Can you work these out from the model? Positions are in its coordinate system, mm. Coordinates: 2 decimals unless noted, no trailing zeros. Write each question's results on one line, items separated by ' | '. Start each with the question number.
```python
from build123d import *
from build123d.topology import SkipClean

# Parameters (mm, degrees)
SKETCH3_R               = 3.175
SKETCH3_R_2             = 1.5875
BOSS_EXTRUDE1_DEPTH     = 127
LPATTERN1_COUNT         = 2
LPATTERN1_PITCH         = 6.6675
BOSS_EXTRUDE2_DEPTH     = 127
CUT_EXTRUDE1_DEPTH      = 128.223842042
CUT_EXTRUDE1_DEPTH_BACK = 128.223842042


with BuildPart() as part:
    # Sketch3 → Boss-Extrude1 (new, symmetric)
    with BuildSketch(Plane(origin=(0, 0, 0), x_dir=(0, 0, -1), z_dir=(1, 0, 0))):
        with Locations((3.33375, 0)):
            Circle(SKETCH3_R)
        with Locations((3.33375, 0)):
            Circle(SKETCH3_R_2, mode=Mode.SUBTRACT)
    extrude(amount=BOSS_EXTRUDE1_DEPTH, both=True)


with BuildPart() as lpattern1_1:
    # LPattern1: pattern copy
    add(part.part.moved(Location(Vector(0, 0, 1) * (1 * LPATTERN1_PITCH))))


with BuildPart() as part_1:
    add(part.part)

    add(lpattern1_1.part)  # Boss-Extrude2 merges LPattern1_1
    # Sketch4 → Boss-Extrude2 (add, symmetric)
    with BuildSketch(Plane(origin=(0, 0, 0), x_dir=(0, 0, -1), z_dir=(1, 0, 0))):
        with BuildLine():
            Line((6.588125, 0.238125), (6.746875, 0.238125))
            ThreePointArc((6.746875, 0.238125), (6.811551474, 0.262993637), (6.842905738, 0.324786885))
            Line((6.842905738, 0.324786885), (6.842905738, -0.324786885))
            ThreePointArc((6.842905738, -0.324786885), (6.811551474, -0.262993637), (6.746875, -0.238125))
            Line((6.746875, -0.238125), (6.588125, -0.238125))
            ThreePointArc((6.588125, -0.238125), (6.523448526, -0.262993637), (6.492094262, -0.324786885))
            Line((6.492094262, -0.324786885), (6.492094262, 0.324786885))
            ThreePointArc((6.492094262, 0.324786885), (6.523448526, 0.262993637), (6.588125, 0.238125))
        make_face()
        with BuildLine():
            Line((0.175405738, 0.324786885), (0.175405738, -0.324786885))
            ThreePointArc((0.175405738, -0.324786885), (0.144051474, -0.262993637), (0.079375, -0.238125))
            Line((0.079375, -0.238125), (-0.079375, -0.238125))
            ThreePointArc((-0.079375, -0.238125), (-0.144051474, -0.262993637), (-0.175405738, -0.324786885))
            Line((-0.175405738, -0.324786885), (-0.175405738, 0.324786885))
            ThreePointArc((-0.175405738, 0.324786885), (-0.144051474, 0.262993637), (-0.079375, 0.238125))
            Line((-0.079375, 0.238125), (0.079375, 0.238125))
            ThreePointArc((0.079375, 0.238125), (0.144051474, 0.262993637), (0.175405738, 0.324786885))
        make_face()
    extrude(amount=BOSS_EXTRUDE2_DEPTH, both=True)

    # Sketch5 → Cut-Extrude1 (cut, two sides: drawn at the far end of the back side and taken through both)
    with SkipClean():  # the faces are left unmerged after this step: merging them gives an invalid solid
        with BuildSketch(Plane(origin=(0, 0, 0), x_dir=(0, 0, -1), z_dir=(1, 0, 0)).offset(-CUT_EXTRUDE1_DEPTH_BACK)):
            with BuildLine():
                Line((6.492094262, 0.324786885), (6.842905738, 0.324786885))
                Line((6.842905738, 0.324786885), (6.842905738, -0.324786885))
                Line((6.842905738, -0.324786885), (6.492094262, -0.324786885))
                ThreePointArc((6.492094262, -0.324786885), (6.50875, 0), (6.492094262, 0.324786885))
            make_face()
        extrude(amount=CUT_EXTRUDE1_DEPTH + CUT_EXTRUDE1_DEPTH_BACK, mode=Mode.SUBTRACT)


solid = part_1.part
```
Q1. I need wall thicknesses on line 1 along Y through (x, z) = (-42, 3.25); line 2 along Z through (x, y) = (85.5, -0.75); line 3 along Y through (x, z) = (14, 2.25). Which ranges of each line are inside material? Lowest first, please. Write a range as from..to.
Q2. If we section it at A-A (x = 85.5): Count the separate pieces of the cut face and the enclosed holes in it, then the cut area to 3 significant figures.
Q3. I'm going to push flat-ended pins straight in: pin 1 Ø1.5 at (x, y) = (20.5, 2) entering from -Z; pin 2 Ø2 at (x, y) = (78, -2) entering from +Z. Where does each tip first touch, or does it pass through?
Q4. Thinking about a two-plate mould opening in Z: for faces 1 (the face through (1.778, 0.135, 6.506)), 2 (the face through (127, 0, 0)), which applies, pulls with the +Z half, pulls with the -Z half, needs draft (parallel to the pull), parting line crosses it, or undercut?
Answer list:
1) line 1: y = -3.17..-1.59, 1.59..3.17 | line 2: z = -6.42..-4.73, -1.93..-0.25, 0.25..1.93, 4.73..6.42 | line 3: y = -2.98..-1.16, 1.16..2.98
2) separate pieces: 1 | enclosed holes: 2 | area: 47.7 mm2
3) pin 1: stops at z = -6.25 | pin 2: stops at z = 6.35
4) face 1: undercut | face 2: needs draft
